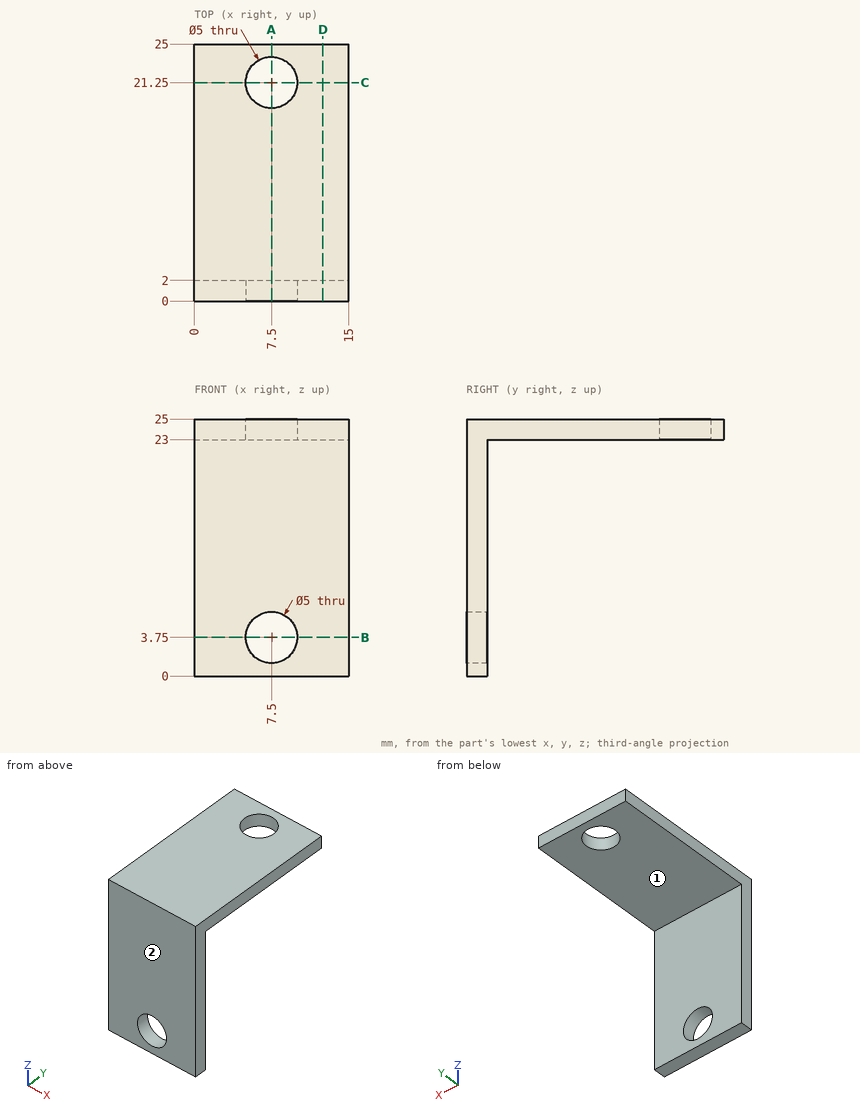
The figure shows three views and two pictorial views of one solid part (mm, origin at its lowest corner). Answer the questions. A direction names the side the tool comes from. Coordinates: 2 decimals unless noted, no trailing zeros. Order: outer loops, then holes, each group sorted by start corner. A loop starts at its lowest first (then second) coordinate and runs counter-clockwise, first axis right, second up.
Q1. A cutting plane is placed at C-C, the plane y = 21.25. Write down the section's boundary in (x, z).
Q2. A cutting plane is placed at A-A, the plane x = 7.5. Write down the section's boundary in (y, z), and give its area (3 significant figures).
Q3. A cutting plane is placed at D-D, the plane x = 12.5. Write down the section's boundary in (y, z).
Q4. Which of the six approach directions +Z, -Z, +X, -X, +Y, -Y give full straight-line access (tool end or side, diameter ignored) to the marked faces 1 and 2?
Q5. Given P1, Ø5, axis at x = 12.5, z = 8.5, coming from the +Y side; P2, Ø7.5, axis at x = 4, y = 13.5, coming from the -Z side; P3, Ø4.5, axis at x = 7.5, z = 3.75, coming from the -Y side, each flat-ended and moving along its own axis, determine where each tip first touches the part or whether it passes through.
Q6. Consider line 1 (X direction, y = 0.65, z = 3.75); line 2 (Y direction, x = 7.5, z = 24); line 3 (Y direction, x = 5, z = 20.25). Determine where each line is inside the solid, lowest interval first.
Q7. A cutting plane is placed at B-B, the plane z = 3.75. Write down the section's boundary in (x, y).
Answers follow:
1. outline: (0, 23) - (5, 23) - (5, 25) - (0, 25) - close; (10, 23) - (15, 23) - (15, 25) - (10, 25) - close
2. outline: (0, 0) - (2, 0) - (2, 1.25) - (0, 1.25) - close; (0, 6.25) - (2, 6.25) - (2, 23) - (18.75, 23) - (18.75, 25) - (0, 25) - close; (23.75, 23) - (25, 23) - (25, 25) - (23.75, 25) - close
2. area: 76.0 mm2
3. outline: (0, 0) - (2, 0) - (2, 23) - (25, 23) - (25, 25) - (0, 25) - close
4. face 1: -Z, +X, -X, +Y
4. face 2: +Z, -Z, +X, -X, -Y
5. P1: stops at y = 2
5. P2: stops at z = 23
5. P3: passes through
6. line 1: x = 0 to 5, 10 to 15
6. line 2: y = 0 to 18.75, 23.75 to 25
6. line 3: y = 0 to 2
7. outline: (0, 0) - (5, 0) - (5, 2) - (0, 2) - close; (10, 0) - (15, 0) - (15, 2) - (10, 2) - close
